The drawing under review shows one solid part. Ordinate dimensions are in mm from its lowest x, y, z. Round coordinates to 2 decimals unless told otherwise and drop trailing zeros. Write each loop counter-clockwise with the first axis right and the second up, starting at its lowest first coordinate (ties: lowest second). Pieces come first, ordered by that corner, then holes.
Item 1: Draft analysis for pull direction Z (two halves, no side actions). For the marked faces 1, 2 and 3, state which applies: +Z half, -Z half, draft (parallel to the pull), parting line (faces both ways), or undercut.
Item 2: Add section A-A (y = 5.25). Give the boundary of the cut face in (x, z), plus the area to 3 significant figures.
Item 3: Clearance check with flat-ended pins moving along their axes: pin 1 Ø1 at (y, z) = (2, 24.5) entering from +X; pin 2 Ø1 at (x, y) = (27, 9.5) entering from -Z; pin 3 Ø4 at (x, y) = (14, 9.5) entering from +Z (1 decimal). State where each tip first meets the part, or that it passes through.
Item 4: To check wall thickness, follow L1, parallel to Z at x = 36, y = 11.25 (1 decimal); L2, parallel to Z at x = 58, y = 12.25 (1 decimal); L3, parallel to X at y = 12.25, z = 24 (1 decimal). State the ranges of each line that lie inside material, in increasing order.
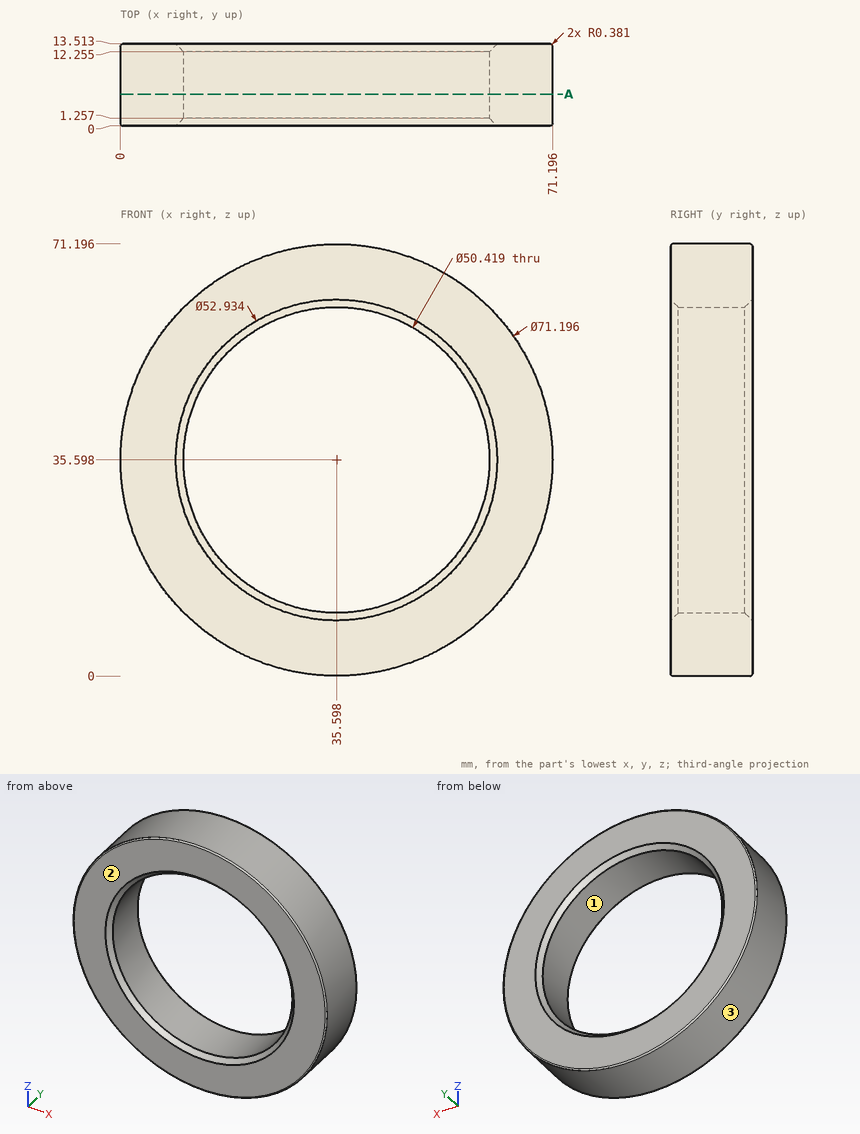
Numbers:
1. face 1: undercut
1. face 2: draft
1. face 3: parting line
2. outline: circle Ø71.2 at (35.6, 35.6); hole circle Ø50.42 at (35.6, 35.6)
2. area: 1,980 mm2
3. pin 1: stops at x = 69.58
3. pin 2: stops at z = 0.93
3. pin 3: stops at z = 65.3
4. L1: z = 0 to 10.4, 60.8 to 71.2
4. L2: z = 7.9 to 24, 47.2 to 63.3
4. L3: x = 1.9 to 13.2, 58 to 69.3
